The listing builds one solid part. Answer for the finished solid, in the listing's coordinates (mm). Face numbers are marked on the shaded views. A direction names the side the tool comes from. Coordinates: 2 decimals unless noted, no trailing zeros. Write each loop counter-clockwise with the first axis right and the second up, starting at its lowest first coordinate (ties: lowest second). Pieces come first, ordered by that corner, then holes.
from build123d import *

# Parameters (mm, degrees)
F0_W      = 50
F0_H      = 50
F0_R      = 2.55
F1_DEPTH  = 3
F2_W      = 20
F2_H      = 20
F3_DEPTH  = 20
F4_W      = 10.1
F4_H      = 10.1
F5_DEPTH  = 25
F7_W      = 10.1
F7_H      = 10.1
F8_DEPTH  = 25
F15_W     = 10.1
F15_H     = 10.1
F16_DEPTH = 25


with BuildPart() as f1:
    # F0 (on Top) → F1 (new body)
    with BuildSketch(Plane.XY):
        Rectangle(F0_W, F0_H)
        Circle(F0_R, mode=Mode.SUBTRACT)
    extrude(amount=F1_DEPTH)

    # F2 (on face) → F3 (join)
    with BuildSketch(Plane.XY.offset(3)):
        Rectangle(F2_W, F2_H)
    extrude(amount=F3_DEPTH)

    # F4 (on Right) → F5 (cut)
    with BuildSketch(Plane.YZ):
        with Locations((0, 13)):
            Rectangle(F4_W, F4_H)
    extrude(amount=-F5_DEPTH, mode=Mode.SUBTRACT)

    # F7 (on 3pt) → F8 (cut)
    with BuildSketch(Plane(origin=(0, 0, 0), x_dir=(-0.7071067812, 0.7071067812, 0), z_dir=(0.7071067812, 0.7071067812, 0))):
        with Locations((0, 13)):
            Rectangle(F7_W, F7_H)
    extrude(amount=F8_DEPTH, mode=Mode.SUBTRACT)

    # F15 (on line) → F16 (cut)
    with BuildSketch(Plane(origin=(4.3333333333, -4.3333333333, 4.3333333333), x_dir=(-0.8164965809, -0.4082482905, 0.4082482905), z_dir=(-0.5773502692, 0.5773502692, -0.5773502692))):
        with Locations((5.307227776, 9.1923881554)):
            Rectangle(F15_W, F15_H)
    extrude(amount=-F16_DEPTH, mode=Mode.SUBTRACT)


solid = f1.part
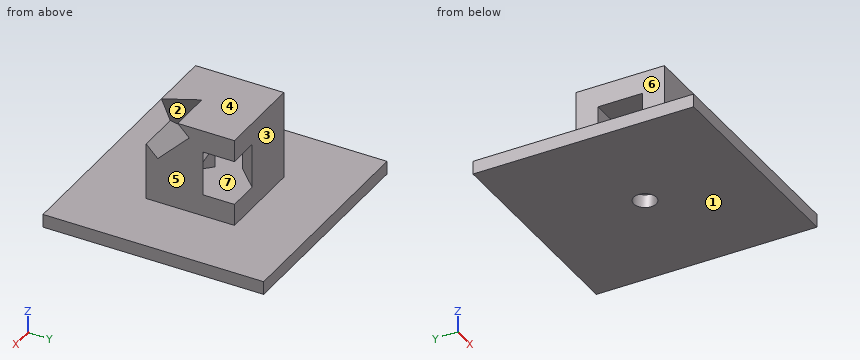
Q1. Determine the mould class of the marked faces 1, 2, 3 and 4 for opening direction Z: released by +Z, released by -Z, zero draft, split by the parting line, or undercut.
Answers below:
face 1: released by -Z
face 2: undercut
face 3: zero draft
face 4: released by +Z
Q2. Which of the six approach directions +Z, -Z, +X, -X, +Y, -Y give full straight-line access (tool end or side, diameter ignored) to the marked faces 5, 6 and 7?
Answers below:
face 5: +Z, +X, +Y, -Y
face 6: +Z, -X, +Y, -Y
face 7: none
Q3. The part is cut by section A-A, the plane x = -5. Write down the section's boundary in (y, z).
Answers below:
outline: (-25, 0) - (25, 0) - (25, 3) - (10, 3) - (10, 23) - (-10, 23) - (-10, 3) - (-25, 3) - close; hole (-5.05, 7.95) - (5.05, 7.95) - (5.05, 18.05) - (-5.05, 18.05) - close
Q4. Find the intervals of material crossed by probe 1 along Y at (x, z) = (0, 1.7); probe 2 along Z at (x, y) = (-9, -2); probe 3 along Z at (x, y) = (11.5, -7), in increasing order.
Answers below:
probe 1: y = -25 to -2.55, 2.55 to 25
probe 2: z = 0 to 7.95, 18.05 to 23
probe 3: z = 0 to 3
Q5. Given pin 1 (7.5 mm diameter, centred on x = 2, y = 3, fed in from -Z); pin 2 (1.5 mm diameter, centred on x = -1.5, z = 10.5, fed in from +Y); pin 3 (3 mm diameter, centred on x = 12.5, y = -16.5, fed in from +Z); pin 4 (6 mm diameter, centred on x = -3, z = 13.5, fed in from -Y), each flat-ended and moving along its own axis, determine where each tip first touches the part or whether it passes through.
Answers below:
pin 1: stops at z = 0
pin 2: stops at y = 10
pin 3: stops at z = 3
pin 4: stops at y = -10
Q6. The part is cut by section C-C, the plane x = -11. Write down the section's boundary in (y, z).
Answers below:
outline: (-25, 0) - (25, 0) - (25, 3) - (-25, 3) - close
Q7. The part is cut by section B-B, the plane z = 4.75. Write down the section's boundary in (x, y).
Answers below:
outline: (-10, -10) - (10, -10) - (10, 10) - (-10, 10) - close
